```python
from build123d import *

# Parameters (mm, degrees)
BOSS_EXTRUDE1_DEPTH = 1
CIRPATTERN1_COUNT   = 2
CIRPATTERN1_ANGLE   = 90


with BuildPart() as part:
    # Sketch2 → Boss-Extrude1 (new body)
    with BuildSketch(Plane(origin=(0, 0, 0), x_dir=(1, 0, 0), z_dir=(0, 1, 0))):
        with BuildLine():
            Line((-5, 0), (-5, -7.5))
            Line((-5, -7.5), (5, -7.5))
            Line((5, -7.5), (5, 0))
            ThreePointArc((5, 0), (0, 5), (-5, 0))
        make_face()
        with BuildLine():
            Line((2.075, 0.425), (2.075, -0.425))
            ThreePointArc((2.075, -0.425), (0, -2.5), (-2.075, -0.425))
            Line((-2.075, -0.425), (-2.075, 0.425))
            ThreePointArc((-2.075, 0.425), (0, 2.5), (2.075, 0.425))
        make_face(mode=Mode.SUBTRACT)
    boss_extrude1 = extrude(amount=BOSS_EXTRUDE1_DEPTH)

    # CirPattern1: Boss-Extrude1 ×2 about axis
    cirpattern1_axis = Axis((-5, 1, 7.5), (1, 0, 0))
    for i in range(1, CIRPATTERN1_COUNT):
        add(boss_extrude1.rotate(cirpattern1_axis, i * CIRPATTERN1_ANGLE / (CIRPATTERN1_COUNT - 1)))


solid = part.part
```
Could you check a few things on this model? Use its own coordinates, in mm. A direction names the side the tool comes from. Give positions to 0.01 mm unless a question says otherwise; leave off trailing zeros. Write each loop counter-clockwise with the first axis right and the second up, starting at its lowest first coordinate (ties: lowest second). Pieces come first, ordered by that corner, then holes. Notation, with made-up numbers: (69.25, 68) - (82.25, 68) arc R15 ccw to (82.25, 75) - close; hole circle Ø3 at (-10, -27). An arc over 180 degrees is marked (long way). One line per item, written item: value. Start each with the question number.
Item 1: I'm going to push flat-ended pins straight in: pin 1 (5 mm diameter, centred on x = -4, z = 1, fed in from -Y); pin 2 (2 mm diameter, centred on x = -2, z = 3, fed in from +Y); pin 3 (1 mm diameter, centred on x = -3.5, y = 6, fed in from -Z). Where does each tip first touch, or does it pass through?
Item 2: Please list where these lines run through material, in increasing order: line 1 (Y direction, x = -2.5, z = 4.5); line 2 (Z direction, x = 1.25, y = 12.5); line 3 (X direction, y = 10, z = 7). Write a range as from..to.
Item 3: If we mould it in two halves opening along Z, with no side actions, what happens to faces 4 (the face through (1, 6, 6.5)), 5 (the face through (-2.075, 0.5, 0)), 6 (the face through (0, 0, 3)), 7 (the face through (0, 0.5, 2.5))? For each: +Z half, -Z half, draft (parallel to the pull), parting line (faces both ways), or undercut.
Item 4: Imagine slicing it at C-C, the plane z = 2. List the corners of the cut face in (x, y) for me, and give its area (3 significant figures).
Item 5: Imagine slicing it at D-D, the plane x = -4. List the corners of the cut face in (y, z) for me, and give its area (3 significant figures).
Item 6: Imagine slicing it at A-A, the plane x = 0. List the corners of the cut face in (y, z) for me, and give its area (3 significant figures).
Item 7: Imagine slicing it at B-B, the plane y = 7.75. List the corners of the cut face in (x, z) for me, and give its area (3 significant figures).
Item 8: Which directions (+Z, -Z, +X, -X, +Y, -Y) give clear straight access to the entire face, cutting with the end or side of a thin tool? Please do faces 1 (the face through (0, 6, 7)), 2 (the face through (2.075, 0.5, 0)), 3 (the face through (0, 1, 3)).
Geometry says:
1. pin 1: y = 0
1. pin 2: y = 1
1. pin 3: z = 6.5
2. line 1: 0..1
2. line 2: 6.5..7.5
2. line 3: -4.77..-1.77, 1.77..4.77
3. face 4: -Z half
3. face 5: undercut
3. face 6: draft
3. face 7: undercut
4. outline: (-5, 0) - (-1.35, 0) - (-1.35, 1) - (-5, 1) - close; (1.35, 0) - (5, 0) - (5, 1) - (1.35, 1) - close
4. area: 7.30 mm^2
5. outline: (0, -3) - (1, -3) - (1, 6.5) - (11.5, 6.5) - (11.5, 7.5) - (0, 7.5) - close
5. area: 21.0 mm^2
6. outline: (0, -5) - (1, -5) - (1, -2.5) - (0, -2.5) - close; (0, 2.5) - (1, 2.5) - (1, 6.5) - (6, 6.5) - (6, 7.5) - (0, 7.5) - close; (11, 6.5) - (13.5, 6.5) - (13.5, 7.5) - (11, 7.5) - close
6. area: 15.0 mm^2
7. outline: (-5, 6.5) - (-2.05, 6.5) - (-2.05, 7.5) - (-5, 7.5) - close; (2.05, 6.5) - (5, 6.5) - (5, 7.5) - (2.05, 7.5) - close
7. area: 5.90 mm^2
8. face 1: +Z, -Z
8. face 2: +Y, -Y
8. face 3: -Z, +X, -X, +Y
